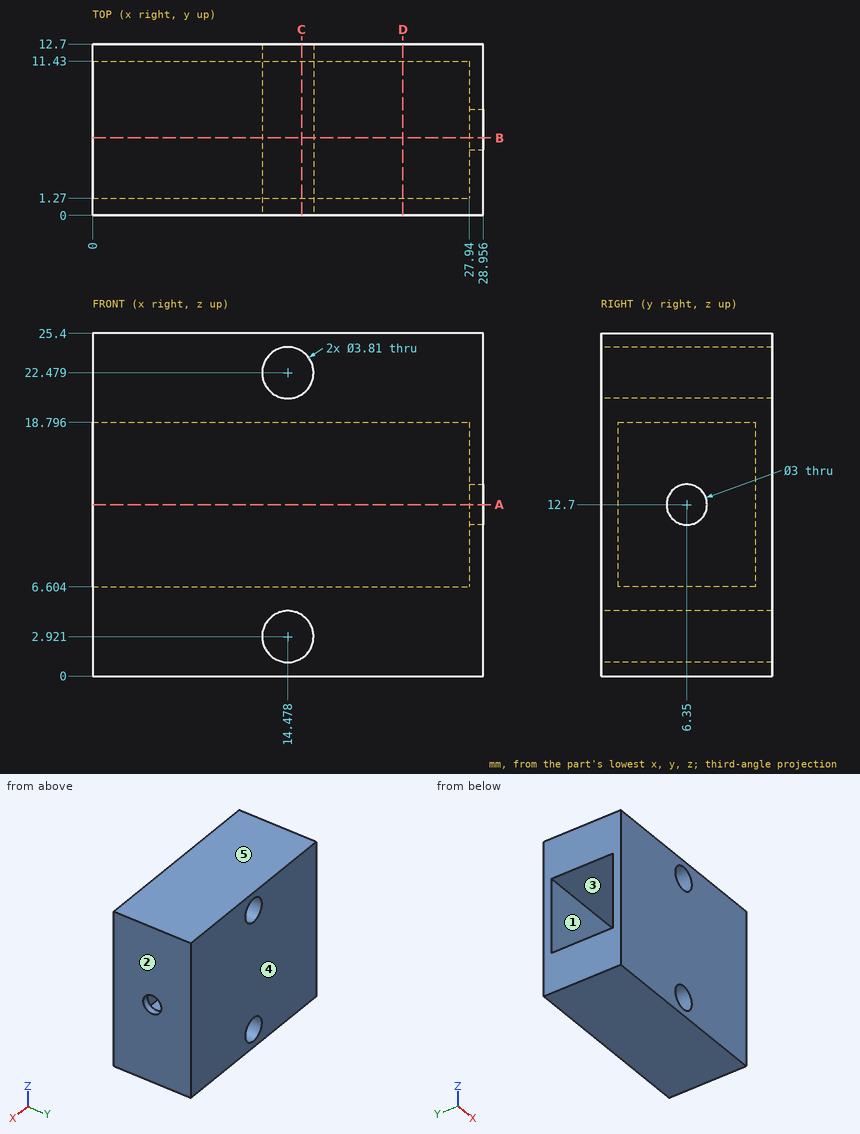
Could you check a few things on this drawing? It's one solid part, dimensions in mm from its lowest x, y, z. A direction names the side the tool comes from. Coordinates: 2 decimals unless noted, no trailing zeros. Loops run counter-clockwise (first coordinate to the right, second up) from the corner with the lowest first, then second, coordinate; pieces in that order, holes last. Notation, with made-up numbers: (61.5, -17.5) - (96.5, -17.5) arc R8 ccw to (96.5, -13.5) - close; hole circle Ø3 at (69, 27.5). An arc over 180 degrees is marked (long way). Return JSON: item names as keys, results as strings. Group by question number.
Item 1: If we section it at D-D on x = 23: Write out the boundary of the cut face in (y, z).
Item 2: On a 3-axis mill with a long thin cutter (end or side, diameter ignored), from which of +Z, -Z, +X, -X, +Y, -Y can I reach the whole of each face in a straight line? I mean the marked faces 1 and 2. Say none if no direction works.
Item 3: If we section it at A-A on z = 12.7: Write out the boundary of the cut face in (x, y).
Item 4: I need wall thicknesses on line 1 (Y direction, x = 13.5, z = 9.25); line 2 (Z direction, x = 17, y = 4); line 3 (X direction, y = 7.25, z = 18.5). Which ranges of each line are inside material? Lowest first, please. Write a range as from..to.
Item 5: If we section it at B-B on y = 5.75: Write out the boundary of the cut face in (x, z) (3 decimals), and give its area (3 significant figures).
Item 6: If we section it at C-C on x = 15.5: Write out the boundary of the cut face in (y, z), and give its area (3 significant figures).
Item 7: Will these pins go through, and if not, where does the flat tip stop? P1, Ø2.5, axis at y = 6.35, z = 12.7, coming from the +X side; P2, Ø3, axis at y = 6.5, z = 15, coming from the -X side.
Item 8: We'd pull the mould along Y, two halves only. Please class the marked faces 3, 4 and 5: +Y half, -Y half, draft (parallel to the pull), parting line (faces both ways), or undercut.
Calculated:
{
 "1": {"outline": "(0, 0) - (12.7, 0) - (12.7, 25.4) - (0, 25.4) - close; hole (1.27, 6.6) - (11.43, 6.6) - (11.43, 18.8) - (1.27, 18.8) - close"},
 "2": {"face 1": "-X", "face 2": "+Z, -Z, +X, +Y, -Y"},
 "3": {"outline": "(0, 0) - (28.96, 0) - (28.96, 4.85) - (27.94, 4.85) - (27.94, 1.27) - (0, 1.27) - close; (0, 11.43) - (27.94, 11.43) - (27.94, 7.85) - (28.96, 7.85) - (28.96, 12.7) - (0, 12.7) - close"},
 "4": {"line 1": "y = 0..1.27, 11.43..12.7", "line 2": "z = 0..6.6, 18.8..25.4", "line 3": "x = 27.94..28.96"},
 "5": {"outline": "(0, 0) - (28.956, 0) - (28.956, 11.325) - (27.94, 11.325) - (27.94, 6.604) - (0, 6.604) - close; (0, 18.796) - (27.94, 18.796) - (27.94, 14.075) - (28.956, 14.075) - (28.956, 25.4) - (0, 25.4) - close; hole circle Ø3.81 at (14.478, 2.921); hole circle Ø3.81 at (14.478, 22.479)", "area": "369 mm^2"},
 "6": {"outline": "(0, 0) - (12.7, 0) - (12.7, 1.31) - (0, 1.31) - close; (0, 4.53) - (12.7, 4.53) - (12.7, 20.87) - (0, 20.87) - close; (0, 24.09) - (12.7, 24.09) - (12.7, 25.4) - (0, 25.4) - close; hole (1.27, 6.6) - (11.43, 6.6) - (11.43, 18.8) - (1.27, 18.8) - close", "area": "117 mm^2"},
 "7": {"P1": "passes through", "P2": "stops at x = 27.94"},
 "8": {"face 3": "undercut", "face 4": "+Y half", "face 5": "draft"}
}
